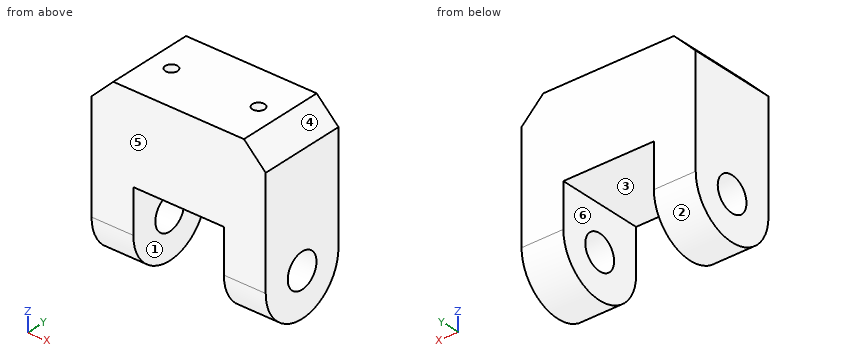
Autodesk Inventor part; units mm, degrees
ref_plane "YZ Plane" through (0, 0, 0) normal (1, 0, 0) x (0, 1, 0)
ref_plane "XZ Plane" through (0, 0, 0) normal (0, 1, 0) x (-1, 0, 0)
ref_plane "XY Plane" through (0, 0, 0) normal (0, 0, 1) x (1, 0, 0)
sketch "Sketch1" plane through (0, 0, 0) normal (1, 0, 0) x (0, 1, 0)
  line L0 (4.6679, 5.5772) -> (-8.0321, 5.5772)
  line L1 (-8.0321, 5.5772) -> (-8.0321, -13.4728)
  line L2 (-1.6821, -19.8228) -> (-1.6821, -19.8228)
  line L3 (4.6679, -13.4728) -> (4.6679, 5.5772)
  circle A0 centre (-1.6821, -13.4728) radius 2.5083
  arc A1 (-1.6821, -19.8228) -> (4.6679, -13.4728) centre (-1.6821, -13.4728) ccw
  arc A2 (-8.0321, -13.4728) -> (-1.6821, -19.8228) centre (-1.6821, -13.4728) ccw
  point P0 (0, 0)
  point P1 (-8.0321, -19.8228)
  point P2 (4.6679, -19.8228)
  dimension "d0" = 12.7
  dimension "d1" = 25.4
  dimension "d2" = 5.0165
  dimension "d3" = 6.35
  dimension "d4" = 6.35
extrude "Extrusion1" add sketch "Sketch1" against normal blind 25.4
sketch "Sketch2" plane through (0, -8.0321, 5.5772) normal (0, 0, 1) x (1, 0, 0)
  line L0 (0, 0) -> (-25.4, 0)
  line L1 (0, 12.7) -> (0, 0)
  circle A0 centre (-6.35, 6.35) radius 0.889
  circle A1 centre (-19.05, 6.35) radius 0.889
  line L2 (-25.4, 0) -> (-25.4, 12.7)
  point P0 (0, 8.0321)
  point P1 (-12.7, 6.35)
  dimension "d7" = 6.35
  dimension "d8" = 12.7
  dimension "d9" = 1.778
  dimension "d10" = 6.35
  dimension "d11" = 1.778
  dimension "d12" = 6.35
extrude "Extrusion2" cut sketch "Sketch2" against normal blind 11.43
chamfer "Chamfer1" distance 3.175 angle 45 2 edges at (0, -1.6821, 5.5772) (-25.4, -1.6821, 5.5772)
sketch "Sketch3" plane through (-25.4, 4.6679, -13.4728) normal (0, 1, 0) x (1, 0, 0)
  line L0 (25.4, 6.35) -> (0, 6.35)
  line L1 (6.096, 6.35) -> (19.304, 6.35)
  line L2 (19.304, 6.35) -> (19.304, -6.35)
  line L3 (19.304, -6.35) -> (6.096, -6.35)
  line L4 (6.096, -6.35) -> (6.096, 6.35)
  line L5 (25.4, 0) -> (25.4, 6.35)
  line L6 (0, 6.35) -> (0, 0)
  point P0 (25.4, -13.4728)
  dimension "d18" = 12.7
  dimension "d19" = 6.096
  dimension "d20" = 6.096
extrude "Extrusion3" cut sketch "Sketch3" against normal blind 12.7
properties part number "band_hinge"
Part model, mm, in its own coordinate system. Face numbers are marked on the shaded views. A direction names the side the tool comes from. Give positions to 0.01 mm unless a question says otherwise; leave off trailing zeros. Loops run counter-clockwise (first coordinate to the right, second up) from the corner with the lowest first, then second, coordinate; pieces in that order, holes last. Notation, with made-up numbers: (63, 55) -> (96, 55) arc R14 ccw to (96, 79) -> close; hole circle Ø3 at (-9.75, -4). An arc over 180 degrees is marked (long way). Write each question's results on one line, items separated by ' | '. Start each with the question number.
Q1. Pull direction X, two halves, no side cores. Call the marked faces 3, 4, 5 and 6: +X half, -X half, draft (parallel to the pull), parting line (faces both ways), or undercut.
Q2. Band-saw the part on D-D on x = -12.5. List the corners of the cut face in (y, z), plus the area to 3 significant figures.
Q3. Band-saw the part on B-B on y = 0.5. List the corners of the cut face in (x, z) (3 decimals), plus the area to 3 significant figures.
Q4. Wall check: L1, parallel to X at y = -1, z = 3.5; L2, parallel to X at y = 0, z = -18.75; L3, parallel to X at y = -1.5, z = 4. Give the ranges that are in metal, low to high.
Q5. Which spindle directions (+Z, -Z, +X, -X, +Y, -Y) get a long thin tool onto all of the face, cutting with end or side? Do the marked faces 1 and 2. Say none if no direction does.
Q6. Pin check, flat tips, straight feed: P1, Ø0.9, axis at x = -19, y = -1.5, coming from the +Z side; P2, Ø1, axis at x = -11.5, y = -6, coming from the -Z side. Stop position of each tip, or through.
Q7. Band-saw the part on C-C on x = -23. List the corners of the cut face in (y, z), plus the area to 3 significant figures.
Q8. Band-saw the part on A-A on z = -9.5. List the corners of the cut face in (x, y), plus the area to 3 significant figures.
Results are:
1) face 3: undercut | face 4: +X half | face 5: draft | face 6: undercut
2) outline: (-8.03, -7.12) -> (4.67, -7.12) -> (4.67, 5.58) -> (-8.03, 5.58) -> close | area: 161 mm²
3) outline: (-25.4, -19.436) -> (-19.304, -19.436) -> (-19.304, -14.71) -> (-25.4, -14.71) -> close; (-25.4, -12.236) -> (-19.304, -12.236) -> (-19.304, -7.123) -> (-6.096, -7.123) -> (-6.096, -12.236) -> (0, -12.236) -> (0, 2.402) -> (-3.175, 5.577) -> (-22.225, 5.577) -> (-25.4, 2.402) -> close; (-6.096, -19.436) -> (0, -19.436) -> (0, -14.71) -> (-6.096, -14.71) -> close | area: 432 mm²
4) L1: x = -24.3 to -19.62, -18.48 to -6.92, -5.78 to -1.1 | L2: x = -25.4 to -19.3, -6.1 to 0 | L3: x = -23.8 to -19.92, -18.18 to -7.22, -5.48 to -1.6
5) face 1: -Z, +Y, -Y | face 2: -Z, +X, -X
6) P1: stops at z = -5.85 | P2: stops at z = -7.12
7) outline: (-8.03, -13.47) arc R6.35 ccw to (4.67, -13.47) -> (4.67, 4.8) -> (-8.03, 4.8) -> close; hole circle Ø5.02 at (-1.68, -13.47) | area: 276 mm²
8) outline: (-25.4, -8.03) -> (-19.3, -8.03) -> (-19.3, 4.67) -> (-25.4, 4.67) -> close; (-6.1, -8.03) -> (0, -8.03) -> (0, 4.67) -> (-6.1, 4.67) -> close | area: 155 mm²
